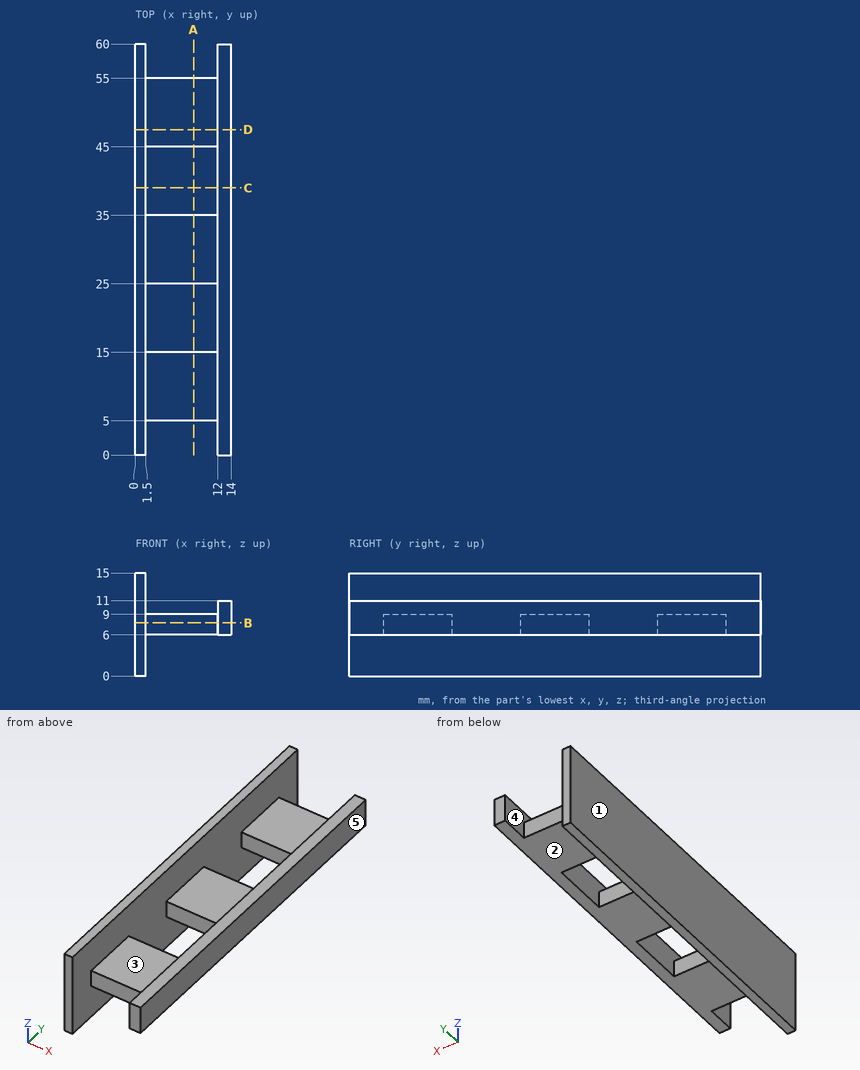
Study the drawing (mm; zero at the part's minimum x, y, z) and answer. A direction names the side the tool comes from. Round coordinates to 2 decimals unless told otherwise and drop trailing zeros. Order: outer loops, then holes, each group sorted by start corner. A loop starts at its lowest first (then second) coordinate and runs counter-clockwise, first axis right, second up. Notation, with made-up numbers: (10, 7) -> (64, 7) arc R6 ccw to (64, 11) -> close; hole circle Ø4 at (-35, 11). An arc over 180 degrees is marked (long way). Answer as CSV lines item,"result". Start each with the question number.
(1) Find the intervals of material crossed by probe 1 along Y at (x, z) = (6.25, 8.5); probe 2 along X at (y, z) = (8.5, 10); probe 3 along Z at (x, y) = (12.75, 27.5), in increasing order. Write a range as from..to.
(2) The part is cut by section C-C (y = 39). Determine the outline of the cut face in (x, z), then the cut area to 3 significant figures.
(3) The part is cut by section D-D (y = 47.5). Determine the outline of the cut face in (x, z).
(4) For a pull along Y with two mould halves and no side action, classify the marked faces 4 and 5 as +Y half, -Y half, draft (parallel to the pull), parting line (faces both ways), or undercut.
(5) The part is cut by section B-B (z = 7.75). Determine the outline of the cut face in (x, y).
(6) Flat-ended cylindrical pins translate along their axes: pin 1 Ø8 at (x, y) = (6.5, 29) entering from +Z; pin 2 Ø6 at (x, z) = (6, 10.5) entering from -Y; pin 3 Ø6 at (x, z) = (6.5, 10.5) entering from +Y. Find the tip coordinate at first contact, or state that the pin passes through.
(7) A tool of negligible diameter and unlimited length cuts with its end or side. For the marked faces 1, 2 and 3, from which of +Z, -Z, +X, -X, +Y, -Y can it reach the whole face along a straight path? Write none if from no direction.
(8) The part is cut by section A-A (x = 8.5). Determine the outline of the cut face in (y, z).
Evaluation:
1,probe 1,"5..15, 25..35, 45..55"
1,probe 2,"0..1.5, 12..14"
1,probe 3,"6..11"
2,outline,"(0, 0) -> (1.5, 0) -> (1.5, 15) -> (0, 15) -> close; (12, 6) -> (14, 6) -> (14, 11) -> (12, 11) -> close"
2,area,"32.5 mm²"
3,outline,"(0, 0) -> (1.5, 0) -> (1.5, 6) -> (14, 6) -> (14, 11) -> (12, 11) -> (12, 9) -> (1.5, 9) -> (1.5, 15) -> (0, 15) -> close"
4,face 4,"undercut"
4,face 5,"draft"
5,outline,"(0, 0) -> (1.5, 0) -> (1.5, 5) -> (12, 5) -> (12, 0) -> (14, 0) -> (14, 60) -> (12, 60) -> (12, 55) -> (1.5, 55) -> (1.5, 60) -> (0, 60) -> close; hole (1.5, 15) -> (12, 15) -> (12, 25) -> (1.5, 25) -> close; hole (1.5, 35) -> (12, 35) -> (12, 45) -> (1.5, 45) -> close"
6,pin 1,"z = 9"
6,pin 2,"y = 5"
6,pin 3,"y = 55"
7,face 1,"+Z, -Z, -X, +Y, -Y"
7,face 2,"-Z, +X, +Y, -Y"
7,face 3,"+Z, +Y, -Y"
8,outline,"(5, 6) -> (15, 6) -> (15, 9) -> (5, 9) -> close; (25, 6) -> (35, 6) -> (35, 9) -> (25, 9) -> close; (45, 6) -> (55, 6) -> (55, 9) -> (45, 9) -> close"
